CAD build for the part. Positions are in the model's coordinates, mm. A direction names the side the tool comes from. Coordinates: 2 decimals unless noted, no trailing zeros. Order: outer loops, then holes, each group sorted by start corner. A loop starts at its lowest first (then second) coordinate and runs counter-clockwise, first axis right, second up. Notation, with made-up numbers: (-35, -1) - (-8, -1) arc R22 ccw to (-8, 7) - close; hole circle Ø5 at (73.25, 18). An arc over 180 degrees is marked (long way). Use one line per item in the form item = value.
```python
from build123d import *

# Parameters (mm, degrees)
SKETCH1_W                    = 32.28
SKETCH1_H                    = 32.28
MAIN_BODY_DEPTH              = 34
SKETCH3_R                    = 3.571875
F_9_32_RIGHT_RAIL_DEPTH      = 1
F_9_32_RIGHT_RAIL_DEPTH_BACK = 8.334375
SKETCH4_R                    = 3.571875
F_9_32_LEFT_RAIL_DEPTH       = 8.334375
SKETCH8_R                    = 3.571875
F_9_32_TOPPER_DEPTH          = 1
F_9_32_TOPPER_DEPTH_BACK     = 10
INNER_START                  = -17.4625
SKETCH13_W                   = 24.987421875
SKETCH13_H                   = 24.987421875
INNER_CAVITY_DEPTH           = 8.73125
INNER_CAVITY_DEPTH_BACK      = 34
HEX_START                    = -17
HEX_HOLE_TOP_DEPTH           = 13.825
TOP_CORNER_REACH             = 36
CUT_EXTRUDE2_DEPTH           = 7.292578
CUT_EXTRUDE3_DEPTH           = 7.292578


with BuildPart() as part:
    # Sketch1 → Main Body (new body)
    with BuildSketch(Plane(origin=(0, 0, 0), x_dir=(1, 0, 0), z_dir=(0, 1, 0))):
        with Locations((16.14, 16.14)):
            Rectangle(SKETCH1_W, SKETCH1_H)
    extrude(amount=MAIN_BODY_DEPTH)

    # Sketch3 → 9/32 Right Rail (cut, two sides)
    with BuildSketch(Plane.XY) as f_9_32_right_rail_sk:
        with Locations((16.14, 17)):
            Circle(SKETCH3_R)
    extrude(amount=F_9_32_RIGHT_RAIL_DEPTH, mode=Mode.SUBTRACT)
    extrude(f_9_32_right_rail_sk.sketch, amount=-F_9_32_RIGHT_RAIL_DEPTH_BACK, mode=Mode.SUBTRACT)

    # Sketch4 → 9/32 Left Rail (cut)
    with BuildSketch(Plane.ZY):
        with Locations((-16.14, 17)):
            Circle(SKETCH4_R)
    extrude(amount=-F_9_32_LEFT_RAIL_DEPTH, mode=Mode.SUBTRACT)

    # Sketch8 → 9/32 Topper (cut, two sides)
    with BuildSketch(Plane(origin=(0, 34, 0), x_dir=(1, 0, 0), z_dir=(0, 1, 0))) as f_9_32_topper_sk:
        with Locations((16.14, 16.14)):
            Circle(SKETCH8_R)
    extrude(amount=F_9_32_TOPPER_DEPTH, mode=Mode.SUBTRACT)
    extrude(f_9_32_topper_sk.sketch, amount=-F_9_32_TOPPER_DEPTH_BACK, mode=Mode.SUBTRACT)

    # Sketch13 → Inner Cavity (cut, two sides)
    with BuildSketch(Plane(origin=(0, 34, 0), x_dir=(1, 0, 0), z_dir=(0, 1, 0)).offset(INNER_START)) as inner_cavity_sk:
        with Locations((19.786289062, 19.786289062)):
            Rectangle(SKETCH13_W, SKETCH13_H)
    extrude(amount=INNER_CAVITY_DEPTH, mode=Mode.SUBTRACT)
    extrude(inner_cavity_sk.sketch, amount=-INNER_CAVITY_DEPTH_BACK, mode=Mode.SUBTRACT)

    # Sketch14 → Hex Hole Top (cut)
    with BuildSketch(Plane(origin=(0, 34, 0), x_dir=(1, 0, 0), z_dir=(0, 1, 0)).offset(HEX_START)):
        Polygon((21.79546875, 19.405186405), (16.14, 22.67037281), (10.48453125, 19.405186405), (10.48453125, 12.874813595), (16.14, 9.60962719), (21.79546875, 12.874813595), align=None)
    extrude(amount=HEX_HOLE_TOP_DEPTH, mode=Mode.SUBTRACT)

    # Sketch16 → Top Corner (cut, up to next)
    with BuildSketch(Plane(origin=(0, 34, 0), x_dir=(1, 0, 0), z_dir=(0, 1, 0)), mode=Mode.PRIVATE) as top_corner_sk1:
        Polygon((32.28, 32.28), (16.276714219, 32.28), (32.28, 16.276714219), align=None)
    top_corner_tool1 = extrude(top_corner_sk1.sketch, amount=-TOP_CORNER_REACH, mode=Mode.PRIVATE) & part.part
    add(top_corner_tool1.solids().sort_by_distance((26.945571, 34, -26.945571))[0], mode=Mode.SUBTRACT)

    # Sketch18 → Cut-Extrude2 (cut)
    with BuildSketch(Plane.ZY):
        Polygon((-32.28, 0), (-16.14, 0), (-32.28, 17), align=None)
    extrude(amount=-CUT_EXTRUDE2_DEPTH, mode=Mode.SUBTRACT)

    # Sketch19 → Cut-Extrude3 (cut)
    with BuildSketch(Plane.XY):
        Polygon((32.28, 0), (16.14, 0), (32.28, 17), align=None)
    extrude(amount=-CUT_EXTRUDE3_DEPTH, mode=Mode.SUBTRACT)


solid = part.part
```
Item 1: Drill centre lines: line 1 (X direction, y = 33, z = -16.14); line 2 (Z direction, x = 9.5, y = 23); line 3 (Z direction, x = 16.14, y = 32.4). Where is each one in solid material? Low to high. Write a range as [from, to].
Derived:
line_1 = [0, 12.57], [19.71, 32.28]
line_2 = [-7.29, 0]
line_3 = [-32.28, -19.71], [-12.57, 0]
Item 2: Cut at A-A, the plane x = 14.5. Write the cut outline in (y, z) (3 decimals).
Derived:
outline = (0, -7.293) - (13.827, -7.293) - (13.827, 0) - (0, 0) - close; (20.173, -7.293) - (25.269, -7.293) - (25.269, -10.556) - (30.825, -10.556) - (30.825, -12.967) - (34, -12.967) - (34, 0) - (20.173, 0) - close; (25.269, -32.28) - (34, -32.28) - (34, -19.313) - (30.825, -19.313) - (30.825, -21.724) - (25.269, -21.724) - close
Item 3: Cut at B-B, the plane y = 26.5. Write the cut outline in (x, z).
Derived:
outline = (0, -32.28) - (16.28, -32.28) - (32.28, -16.28) - (32.28, 0) - (0, 0) - close; hole (10.48, -19.41) - (16.14, -22.67) - (21.8, -19.41) - (21.8, -12.87) - (16.14, -9.61) - (10.48, -12.87) - close
Item 4: Two-plate mould, pull along Y, no slides. Class faces 1 (the face through (18.93, 28.01, -11.22)), 2 (the face through (18.06, 20.01, -3.6)), 3 (the face through (6, 0, -6)), 4 (the face through (12, 34, -16)): +Y half, -Y half, draft (parallel to the pull), parting line (faces both ways), or undercut.
Derived:
face_1 = draft
face_2 = undercut
face_3 = -Y half
face_4 = +Y half
Item 5: Cut at C-C, the plane z = -6.5. Write the cut outline in (x, y), plus the area to 3 significant figures.
Derived:
outline = (0, 0) - (16.14, 0) - (32.28, 17) - (32.28, 34) - (0, 34) - close; hole circle Ø7.14 at (16.14, 17)
area = 920 mm²
Item 6: Cut at D-D, the plane y = 16. Write the cut outline in (x, z), plus the area to 3 significant figures.
Derived:
outline = (0, -31.33) - (7.29, -31.33) - (7.29, -19.57) - (0, -19.57) - close; (0, -12.71) - (7.29, -12.71) - (7.29, -7.29) - (12.71, -7.29) - (12.71, 0) - (0, 0) - close; (19.57, -7.29) - (31.33, -7.29) - (31.33, 0) - (19.57, 0) - close
area = 304 mm²
Item 7: Drop flat-ended pins along their axis: pin 1 (1 mm diameter, centred on y = 26.5, z = -17.5, fed in from +X); pin 2 (8 mm diameter, centred on y = 16.5, z = -16, fed in from +X); pin 3 (9 mm diameter, centred on x = 14.5, z = -14.5, fed in from -Y). Give the stop position or say it passes through.
Derived:
pin_1 = 31.56
pin_2 = 7.29
pin_3 = 25.27
Item 8: 3-axis set-ups, long thin cutter, end or side, ignore diameter. For faces 5 (the face through (7.293, 16, -20)), 6 (the face through (13.273, 28.008, -11.265)), 7 (the face through (12, 17, 0)): which of +Z, -Z, +X, -X, +Y, -Y reach the whole face in a straight line?
Derived:
face_5 = -Z, +X, -Y
face_6 = -Y
face_7 = +Z, +X, -X, +Y, -Y
